Design review of the part built by this model. Coordinates are the model's own, in mm. A direction names the side the tool comes from. Coordinates: 2 decimals unless noted, no trailing zeros. Loops run counter-clockwise (first coordinate to the right, second up) from the corner with the lowest first, then second, coordinate; pieces in that order, holes last. Notation, with made-up numbers: M -21,-9.5 L 16,-9.5 A7 ccw 16,-1.5 Z; hole C -29,50 d8. An arc over 180 degrees is marked long. One line per item, written item: value.
Autodesk Inventor part; units mm, degrees
ref_plane "YZ Plane" through (0, 0, 0) normal (1, 0, 0) x (0, 1, 0)
ref_plane "XZ Plane" through (0, 0, 0) normal (0, 1, 0) x (-1, 0, 0)
ref_plane "XY Plane" through (0, 0, 0) normal (0, 0, 1) x (1, 0, 0)
sketch "Sketch1" plane through (0, 0, 0) normal (0, 0, 1) x (1, 0, 0)
  line L0 (-15, 0) -> (-6.35, 0)
  line L1 (-6.35, 0) -> (-6.35, 15)
  line L2 (-6.35, 15) -> (-7.5, 15)
  line L3 (-7.5, 15) -> (-7.5, 3)
  line L4 (-7.5, 3) -> (-15, 3)
  line L5 (-15, 3) -> (-15, 0)
  line L6 (0, -3) -> (0, 18)
  point P0 (0, 0)
  dimension "d0" = 3
  dimension "d2" = 15
  dimension "d3" = 6.35
  dimension "d4" = 15
  dimension "d17" = 7.5
  dimension "d18" = 1.15
revolve "Revolution1" add sketch "Sketch1" angle 360 about axis through (0, -10, 0) along (0, 1, 0)
sketch "Sketch2" plane through (0, 3, 0) normal (0, 1, 0) x (1, 0, 0)
  point P0 (0, 0)
  point P1 (0.0472, 12)
  point P2 (0, -12)
  dimension "d6" = 12
  dimension "d22" = 12
hole "Hole1" at (0.0472, 3, -12) at (0, 3, 12) direction (0, -1, 0) diameter 3.2 end through all
sketch "Sketch4" plane through (0, 3, 0) normal (0, 1, 0) x (1, 0, 0)
  circle A0 centre (0, 0) radius 15
  circle A1 centre (0, 0) radius 7.5
  circle A2 centre (-55, 0) radius 64
  point P0 (7.6909, 12.8783)
  point P1 (7.5, 0)
  point P2 (7.6909, -12.8783)
  dimension "d23" = 128
  dimension "d24" = 55
extrude "Extrusion2" cut sketch "Sketch4" against normal through all contours A0 A2 picked at (10.8452, -2.4648)
sketch "Sketch6" plane through (0, 3, 0) normal (0, 1, 0) x (1, 0, 0)
  arc A0 (7.6909, 12.8783) -> (7.6909, -12.8783) centre (0, 0) ccw
  circle A1 centre (0, 0) radius 7.5
  line L0 (-6.3443, 4) -> (-15, 4)
  line L1 (-15, 4) -> (-15, -4)
  line L2 (-15, -4) -> (-6.3443, -4)
  line L3 (-6.3443, -4) -> (-6.3443, 4)
  point P0 (-14.4568, -4)
  point P1 (-6.3443, -4)
  point P2 (-14.4568, 4)
  dimension "d32" = 4
  dimension "d33" = 4
extrude "Extrusion3" add sketch "Sketch6" along normal up to surface (12 mm away) contours L0 A1 L2 A0
sketch "Sketch7" plane through (-14.4568, 15, -4) normal (0, 1, 0) x (1, 0, 0)
  circle A0 centre (14.4568, -4) radius 6.35
  line L0 (8.1861, -5) -> (-0.5432, -5)
  line L1 (-0.5432, -5) -> (-0.5432, -3)
  line L2 (-0.5432, -3) -> (8.1861, -3)
  line L3 (8.1861, -3) -> (8.1861, -5)
  arc A1 (0, 0) -> (0, -8) centre (14.4568, -4) ccw
  point P0 (-0.5098, -5)
  point P1 (8.1861, -3)
  point P2 (-0.5098, -3)
  dimension "d27" = 1
  dimension "d28" = 1
extrude "Extrusion4" cut sketch "Sketch7" against normal through all contours A0 L0 A1 L2
sketch "Sketch8" plane through (-14.4568, 3, 4) normal (0, 0, 1) x (1, 0, 0)
  line L0 (0, 0) -> (0, 12)
  line L1 (8.1125, 12) -> (0, 12)
  point P0 (7.0914, 12)
  point P1 (4, 6)
  dimension "d35" = 12
  dimension "d37" = 4
  dimension "d38" = 6
hole "Hole2" at (-10.4568, 9, 4) direction (0, 0, -1) diameter 3.2 end through all
properties part number "BaffleClampWithScrew3Dprint" material "Brass, Soft Yellow"
(1) We need section B-B on z = 12. State the section outline as (x, y) points, then the cut area to 3 significant figures.
Reply:
outline: M -9,0 L -1.6,0 L -1.6,3 L -9,3 Z; M 1.6,0 L 7.86,0 L 7.86,3 L 1.6,3 Z
area: 41.0 mm2
(2) To check wall thickness, follow line 1 along Z through (x, y) = (0, 1.9); line 2 along Z through (x, y) = (-7.5, 12.5); line 3 along X through (y, z) = (9, 2.85). State the ranges of each line that lie inside material, in increasing order. Write a range as [from, to].
Reply:
line 1: z = [-15, -13.6], [-10.4, -6.35], [6.35, 10.4], [13.6, 15]
line 2: z = [-4, -1], [1, 4]
line 3: x = [-14.73, -12.06], [-8.86, -5.67], [5.67, 6.94]
(3) Mouldability with a two-part tool opening along Y and no side actions: class faces 6 (the flat face through (-8.7, 8.9, 4)), 7 (the flat face through (-5, 3, 7)), 8 (the cylindrical face through (-8.895, 9.347, -2.521)) as released by +Y, released by -Y, zero draft, split by the parting line, or undercut.
Reply:
face 6: zero draft
face 7: released by +Y
face 8: undercut
(4) Tool access review of faces 1 (the flat face through (-9, 8, -4)), 2 (the cylindrical face through (-7.154, 1.479, -13.184)), 3 (the cylindrical face through (6.344, 7.605, 0.265)), 4 (the cylindrical face through (7.495, 8.916, -0.271)), 5 (the flat face through (-12, 8, 1)): name each direction out of +Z, -Z, +X, -X, +Y, -Y from which nothing blocks a thin tool from reaching the whole face with its end or side.
Reply:
face 1: -Z, -X, +Y
face 2: -Z, +Y, -Y
face 3: +Y, -Y
face 4: +Y
face 5: -X, +Y, -Y
(5) Insertion check: pin 1 (6 mm diameter, centred on y = 11, z = -9, fed in from +X); pin 2 (4 mm diameter, centred on x = -10.46, y = 9, fed in from +Z); pin 3 (6 mm diameter, centred on x = -4, y = 2, fed in from -Z). Each pin has a flat end and moves straight along its axis. Give the tip position at first contact, or say it passes through.
Reply:
pin 1: stops at x = 4.5
pin 2: stops at z = 4
pin 3: stops at z = -14.97
(6) We need section D-D on y = 11. State the section outline as (x, z) points.
Reply:
outline: M -14.97,-1 A15 ccw -14.46,-4 L -6.34,-4 A7.5 ccw long -6.34,4 L -14.46,4 A15 ccw -14.97,1 L -6.27,1 A6.35 cw long -6.27,-1 Z
(7) We need section A-A on y = 9. State the section outline as (x, z) points.
Reply:
outline: M -14.97,-1 A15 ccw -14.46,-4 L -12.06,-4 L -12.06,-1 Z; M -14.97,1 L -12.06,1 L -12.06,4 L -14.46,4 A15 ccw Z; M -8.86,-4 L -6.34,-4 A7.5 ccw long -6.34,4 L -8.86,4 L -8.86,1 L -6.27,1 A6.35 cw long -6.27,-1 L -8.86,-1 Z
(8) We need section C-C on x = 3.5. State the section outline as (y, z) points, then the cut area to 3 significant figures.
Reply:
outline: M 0,-14.59 L 3,-14.59 L 3,-6.63 L 15,-6.63 L 15,-5.3 L 0,-5.3 Z; M 0,5.3 L 15,5.3 L 15,6.63 L 3,6.63 L 3,14.59 L 0,14.59 Z
area: 87.8 mm2
